```python
from build123d import *
from OCP.BRepFilletAPI import BRepFilletAPI_MakeChamfer

# Parameters (mm, degrees)
SKETCH1_W           = 30
SKETCH1_H           = 58
SKETCH1_W_2         = 22
SKETCH1_H_2         = 5
BOSS_EXTRUDE1_DEPTH = 11
CUT_EXTRUDE2_START  = -49
SKETCH2_W           = 11
SKETCH2_H           = 4
CUT_EXTRUDE2_DEPTH  = 49
SKETCH3_R           = 2.25
BOSS_EXTRUDE2_DEPTH = 5
SKETCH4_R           = 3.5
CUT_EXTRUDE3_DEPTH  = 3
CHAMFER1_SIZE       = 2.5
CHAMFER1_SIZE_2     = 1.25
CHAMFER2_SIZE       = 2
SKETCH6_W           = 39.025206684
SKETCH6_H           = 36
CUT_EXTRUDE5_DEPTH  = 72.874891304


with BuildPart() as part:
    # Sketch1 → Boss-Extrude1 (new body)
    with BuildSketch(Plane(origin=(0, 0, 0), x_dir=(0, 0, -1), z_dir=(1, 0, 0))):
        with Locations((15, 29)):
            Rectangle(SKETCH1_W, SKETCH1_H)
        with Locations((15, 42.5)):
            Rectangle(SKETCH1_W_2, SKETCH1_H_2, mode=Mode.SUBTRACT)
        with Locations((15, 6.5)):
            Rectangle(SKETCH1_W_2, SKETCH1_H_2, mode=Mode.SUBTRACT)
        with Locations((15, 15.5)):
            Rectangle(SKETCH1_W_2, SKETCH1_H_2, mode=Mode.SUBTRACT)
        with Locations((15, 51.5)):
            Rectangle(SKETCH1_W_2, SKETCH1_H_2, mode=Mode.SUBTRACT)
        with Locations((15, 33.5)):
            Rectangle(SKETCH1_W_2, SKETCH1_H_2, mode=Mode.SUBTRACT)
        with Locations((15, 24.5)):
            Rectangle(SKETCH1_W_2, SKETCH1_H_2, mode=Mode.SUBTRACT)
    extrude(amount=BOSS_EXTRUDE1_DEPTH)

    # Sketch2 → Cut-Extrude2 (cut)
    with BuildSketch(Plane(origin=(0, 58, 0), x_dir=(1, 0, 0), z_dir=(0, 1, 0)).offset(CUT_EXTRUDE2_START)):
        with Locations((5.5, 6)):
            Rectangle(SKETCH2_W, SKETCH2_H)
    extrude(amount=CUT_EXTRUDE2_DEPTH, mode=Mode.SUBTRACT)

    # Sketch3 → Boss-Extrude2 (add)
    # profile 1 of 2: a face of its own
    with BuildSketch(Plane(origin=(0, 0, 0), x_dir=(1, 0, 0), z_dir=(0, 1, 0))):
        with BuildLine():
            Line((0, 0), (0, -5.5))
            ThreePointArc((0, -5.5), (5.5, -11), (11, -5.5))
            Line((11, -5.5), (11, 0))
            Line((11, 0), (0, 0))
        make_face()
        with Locations(Location((5.5, -5.5, 0), (0, 0, 270))):
            Circle(SKETCH3_R, mode=Mode.SUBTRACT)
    # profile 2 of 2: a face of its own
    with BuildSketch(Plane(origin=(0, 0, 0), x_dir=(1, 0, 0), z_dir=(0, 1, 0))):
        with BuildLine():
            Line((11, 35.5), (11, 30))
            Line((11, 30), (0, 30))
            Line((0, 30), (0, 35.5))
            ThreePointArc((0, 35.5), (5.5, 41), (11, 35.5))
        make_face()
        with Locations(Location((5.5, 35.5, 0), (0, 0, 270))):
            Circle(SKETCH3_R, mode=Mode.SUBTRACT)
    extrude(amount=BOSS_EXTRUDE2_DEPTH)

    # Sketch4 → Cut-Extrude3 (cut)
    with BuildSketch(Plane(origin=(0, 5, 0), x_dir=(1, 0, 0), z_dir=(0, 1, 0))):
        with Locations(Location((5.5, -5.5, 0), (0, 0, 270))):
            Circle(SKETCH4_R)
        with Locations(Location((5.5, 35.5, 0), (0, 0, 270))):
            Circle(SKETCH4_R)
    extrude(amount=-CUT_EXTRUDE3_DEPTH, mode=Mode.SUBTRACT)

    # Chamfer1
    chamfer1_edges_1 = [part.edges().sort_by_distance(p)[0] for p in [
        (5.5, 2, 2),
    ]]
    chamfer1_side_1 = [part.faces().sort_by_distance(p)[0] for p in [
        (5.5, 2.025, 2),
    ]]
    chamfer1_edges_2 = [part.edges().sort_by_distance(p)[0] for p in [
        (5.5, 2, -39),
    ]]
    chamfer1_side_2 = [part.faces().sort_by_distance(p)[0] for p in [
        (5.5, 2.025, -39),
    ]]
    chamfer1 = BRepFilletAPI_MakeChamfer(part.part.solid().wrapped)
    for e in chamfer1_edges_1:
        chamfer1.Add(CHAMFER1_SIZE - 0.0001, CHAMFER1_SIZE_2 - 0.0001, e.wrapped, chamfer1_side_1[0].wrapped)
    for e in chamfer1_edges_2:
        chamfer1.Add(CHAMFER1_SIZE - 0.0001, CHAMFER1_SIZE_2 - 0.0001, e.wrapped, chamfer1_side_2[0].wrapped)
    add(Compound.cast(chamfer1.Shape()), mode=Mode.REPLACE)  # a hair under: the kernel refuses the full size

    # Chamfer2
    chamfer2_edges = [part.edges().sort_by_distance(p)[0] for p in [
        (5.5, 5, 0),
        (5.5, 5, -30),
        (5.5, 4, -4),
        (5.5, 4, -26),
        (5.5, 9, -26),
        (5.5, 40, -26),
        (5.5, 45, -26),
        (5.5, 13, -26),
        (5.5, 18, -26),
        (5.5, 54, -26),
        (5.5, 49, -26),
        (5.5, 36, -26),
        (5.5, 31, -26),
        (5.5, 22, -26),
        (5.5, 27, -26),
    ]]
    chamfer(chamfer2_edges, length=CHAMFER2_SIZE - 0.0001)  # a hair under: the kernel refuses the full size

    # Sketch6 → Cut-Extrude5 (cut, through all)
    with BuildSketch(Plane.ZY):
        with Locations((-14.453310682, 40)):
            Rectangle(SKETCH6_W, SKETCH6_H)
    extrude(amount=-CUT_EXTRUDE5_DEPTH, mode=Mode.SUBTRACT)


solid = part.part
```
Model file for the job. Use its own axes, mm. A direction names the side the tool comes from. Coordinates: 2 decimals unless noted, no trailing zeros. Order: outer loops, then holes, each group sorted by start corner. A loop starts at its lowest first (then second) coordinate and runs counter-clockwise, first axis right, second up. Notation, with made-up numbers: (-22.75, 15.25) - (20.25, 15.25) arc R20 ccw to (20.25, 21.25) - close; hole circle Ø2 at (43, -29.75). An arc over 180 degrees is marked (long way). Return JSON: item names as keys, results as strings. Group by question number.
1) Flat gauge pins, fed straight in: P1, Ø5.5, axis at x = 3, y = 14.5, coming from the -Z side; P2, Ø4.5, axis at x = 5, z = 7, coming from the +Y side; P3, Ø0.5, axis at x = 4.5, y = 15.5, coming from the +Z side. Where does each tip first touch, or does it go through?
2) Saw through at C-C, the plane x = 5.5. Count the separate pieces of the cut face and the enclosed holes in it, plus the area to 3 significant figures.
3) Saw through at A-A, the plane y = 19. Write the cut outline in (x, z), plus the area to 3 significant figures.
4) Probe line 1 (Z direction, x = 5.5, y = 0.55); line 2 (Y direction, x = 6.25, z = -16); line 3 (Z direction, x = 2.5, y = 12.25). List the from-to ranges inside material, lowest first. Write a range as from..to.
5) Saw through at D-D, the plane x = 9.75. Write the cut outline in (y, z).
6) Saw through at B-B, the plane z = -12. Write the cut outline in (x, y).
7) Tool access for faces 4 (the cylindrical face through (5.654, 4.753, -38.997)), 5 (the flat face through (5, 5, -5)), 6 (the flat face through (5, 13, -16)), 7 (the flat face through (5, 14, 0)): list every direction of +Z, -Z, +X, -X, +Y, -Y with a clear straight run to the whole face (end or side of a thin tool).
8) Mould opens along Y. For faces 1 (the cylindrical face through (5.4, 2.5, -41)), 2 (the flat face through (5, 8, -25)), 3 (the flat face through (6, 5, -40)) say: released by +Y, released by -Y, zero draft, split by the parting line, or undercut.
Values found:
{
 "1": {"P1": "stops at z = -30", "P2": "stops at y = 5", "P3": "stops at z = 0"},
 "2": {"separate pieces": "3", "enclosed holes": "0", "area": "478 mm²"},
 "3": {"outline": "(0, -30) - (11, -30) - (11, -8) - (0, -8) - close; (0, -4) - (11, -4) - (11, 0) - (0, 0) - close", "area": "286 mm²"},
 "4": {"line 1": "z = -41..-37.75, -33.25..3.25, 7.75..11", "line 2": "y = 0..4, 9..13, 18..22", "line 3": "z = -30..-8, -4..0"},
 "5": {"outline": "(0, -38.99) - (5, -38.99) - (5, -32) - (7, -30) - (22, -30) - (22, -8) - (18, -8) - (18, -24) - (16, -26) - (15, -26) - (13, -24) - (13, -8) - (9, -8) - (9, -24) - (7, -26) - (6, -26) - (4, -24) - (4, -6) - (6, -4) - (22, -4) - (22, 0) - (7, 0) - (5, 2) - (5, 8.99) - (0, 8.99) - close"},
 "6": {"outline": "(0, 0) - (11, 0) - (11, 4) - (0, 4) - close; (0, 9) - (11, 9) - (11, 13) - (0, 13) - close; (0, 18) - (11, 18) - (11, 22) - (0, 22) - close"},
 "7": {"face 4": "+Y", "face 5": "+X, -X, +Y", "face 6": "+X, -X", "face 7": "+Z, +X, -X, +Y"},
 "8": {"face 1": "zero draft", "face 2": "undercut", "face 3": "released by +Y"}
}
